CAD build for the part. Positions are in the model's coordinates, mm. Give positions to 0.01 mm unless a question says otherwise; leave off trailing zeros. Order: outer loops, then holes, each group sorted by start corner. A loop starts at its lowest first (then second) coordinate and runs counter-clockwise, first axis right, second up. Notation, with made-up numbers: (4, 8) -> (50, 8) arc R10 cw to (50, 13) -> close; hole circle Ø8 at (7.25, 88.25). An arc over 180 degrees is marked (long way). Use one line per item in the form item = value. Start each with the question number.
1) Probe line 1 (Y direction, x = 6.35, z = 1.15); line 2 (X direction, y = 2.75, z = 1.3); line 3 (X direction, y = 3.75, z = 0.6). List the from-to ranges inside material, lowest first.
2) Cut at B-B, the plane y = 2. Give the cut face in (x, z), and give its area (3 significant figures).
3) Cut at A-A, the plane x = 5.05. Give the cut face in (y, z) (3 decimals).
4) Cut at C-C, the plane z = 0.2. State how many separate pieces and enclosed holes the cut face has, and give its area (3 significant figures).
5) Mould opens along X. For faces 1 (the face through (0.87, -4.9, 0.81)), 2 (the face through (-7.65, 0, 1)), 3 (the face through (0, 0, 1.6)) say: pulls with the +X half, pulls with the -X half, needs draft (parallel to the pull), parting line crosses it, or undercut.
6) Cut at D-D, the plane x = 1.27. Give the cut face in (y, z).
from build123d import *

# Parameters (mm, degrees)
SKETCH_W            = 15.3
SKETCH_H            = 11.6
SKETCH_R            = 1.575
PAD_DEPTH           = 1.6
SKETCH001_R         = 0.5
POCKET_DEPTH        = 0.001
POCKET_DEPTH_BACK   = 1.601
LINEARPATTERN_COUNT = 6
LINEARPATTERN_PITCH = 2.54


with BuildPart() as part:
    # Sketch → Pad (new body)
    with BuildSketch(Plane.XY):
        Rectangle(SKETCH_W, SKETCH_H)
        with Locations((-5.05, 3.4)):
            Circle(SKETCH_R, mode=Mode.SUBTRACT)
        with Locations((5.05, 3.4)):
            Circle(SKETCH_R, mode=Mode.SUBTRACT)
    extrude(amount=PAD_DEPTH)

    # Sketch001 → Pocket (cut, two sides)
    with BuildSketch(Plane.XY) as pocket_sk:
        with Locations((-6.35, -4.6)):
            Circle(SKETCH001_R)
    pocket = extrude(amount=-POCKET_DEPTH, mode=Mode.SUBTRACT) + extrude(pocket_sk.sketch, amount=POCKET_DEPTH_BACK, mode=Mode.SUBTRACT)

    # LinearPattern: Pocket ×6
    with Locations(*[(i * LINEARPATTERN_PITCH, 0, 0) for i in range(1, LINEARPATTERN_COUNT)]):
        add(pocket, mode=Mode.SUBTRACT)


solid = part.part
Result:
q1.line_1 = -5.8 to -5.1, -4.1 to 2.51, 4.29 to 5.8
q1.line_2 = -7.65 to -6.48, -3.62 to 3.62, 6.48 to 7.65
q1.line_3 = -7.65 to -6.59, -3.51 to 3.51, 6.59 to 7.65
q2.outline = (-7.65, 0) -> (-5.77, 0) -> (-5.77, 1.6) -> (-7.65, 1.6) -> close; (-4.33, 0) -> (4.33, 0) -> (4.33, 1.6) -> (-4.33, 1.6) -> close; (5.77, 0) -> (7.65, 0) -> (7.65, 1.6) -> (5.77, 1.6) -> close
q2.area = 19.9 mm²
q3.outline = (-5.8, 0) -> (1.825, 0) -> (1.825, 1.6) -> (-5.8, 1.6) -> close; (4.975, 0) -> (5.8, 0) -> (5.8, 1.6) -> (4.975, 1.6) -> close
q4.separate_pieces = 1
q4.enclosed_holes = 8
q4.area = 157 mm²
q5.face_1 = undercut
q5.face_2 = pulls with the -X half
q5.face_3 = needs draft
q6.outline = (-5.8, 0) -> (-5.1, 0) -> (-5.1, 1.6) -> (-5.8, 1.6) -> close; (-4.1, 0) -> (5.8, 0) -> (5.8, 1.6) -> (-4.1, 1.6) -> close
